Could you check a few things on this model? Use its own coordinates, in mm. A direction names the side the tool comes from. Give positions to 0.01 mm unless a question says otherwise; leave off trailing zeros. Loops run counter-clockwise (first coordinate to the right, second up) from the corner with the lowest first, then second, coordinate; pieces in that order, holes last. Notation, with made-up numbers: (21.5, 30.25) - (51.5, 30.25) arc R27 ccw to (51.5, 59.25) - close; hole circle Ø8 at (3.25, 45.25). An arc over 180 degrees is marked (long way). Write each question's results on one line, items separated by ' | '. Start each with the question number.
1) On a 3-axis mill with a long thin cutter (end or side, diameter ignored), from which of +Z, -Z, +X, -X, +Y, -Y can I reach the whole of each face in a straight line? I mean faces 1 (the face through (-1.349, 4.696, -39.603)), 2 (the face through (-46.157, 4.696, -10.863)), 3 (the face through (-50.61, 3.13, 23.15)). Say none if no direction works.
2) I want a section at B-B, the plane x = -14. Write out the boundary of the cut face in (y, z) (3 decimals).
3) If we mould it in two halves opening along Z, with no side actions, what happens to faces 4 (the face through (4.415, 3.637, 35.794)), 5 (the face through (0.1, 1.59, 34.34)), 6 (the face through (34.804, 4.696, -34.533))? For each: +Z half, -Z half, draft (parallel to the pull), parting line (faces both ways), or undercut.
4) I'm going to push flat-ended pins straight in: pin 1 (2 mm diameter, centred on y = 6, z = -20, fed in from +X); pin 2 (2 mm diameter, centred on x = -50.07, z = 16.76, fed in from +Y); pin 3 (4 mm diameter, centred on y = 4.5, z = -10, fed in from -X); pin 4 (3.5 mm diameter, centred on y = 7, z = 34.5, fed in from -X). Where does each tip first touch, or does it pass through?
5) I want a section at C-C, the plane y = 4.5. Count the separate pieces of the cut face and the enclosed holes in it, and give its area (3 significant figures).
6) I want a section at A-A, the plane z = -37. Write out the boundary of the cut face in (x, y) (3 decimals), and give its area (3 significant figures).
7) If I drill on probe 1 along Z at (x, y) = (-3.5, 2.5); probe 2 along X at (y, z) = (2.5, -1.5); probe 3 along Z at (x, y) = (-18, 2.5), over which ranges is the centre line in solid material (lowest first)? Write a range as [from, to].
from build123d import *

# Parameters (mm, degrees)
BOSS_EXTRUDE1_DEPTH = 9.525
SKETCH3_R           = 1.778
BOSS_EXTRUDE2_DEPTH = 6.35
CUT_EXTRUDE1_DEPTH  = 62.992


with BuildPart() as part:
    # Sketch2 → Boss-Extrude1 (new body)
    with BuildSketch(Plane(origin=(0, 0, 0), x_dir=(1, 0, 0), z_dir=(0, 1, 0))):
        with BuildLine():
            ThreePointArc((-27.371275132, 38.745818095), (-40.973617499, 30.433742494), (-46.191603644, 15.370975839))
            ThreePointArc((-46.191603644, 15.370975839), (-46.156170212, 10.799100226), (-46.01239655, 6.229348451))
            ThreePointArc((-46.01239655, 6.229348451), (-45.554867394, -4.424369785), (-44.211253726, -15.00292108))
            ThreePointArc((-44.211253726, -15.00292108), (-36.72609395, -29.152486681), (-21.949825784, -35.308761743))
            ThreePointArc((-21.949825784, -35.308761743), (4.789142288, -35.769006094), (31.212812312, -31.649066671))
            ThreePointArc((31.212812312, -31.649066671), (41.496738573, -25.613366213), (46.788564963, -14.927609673))
            ThreePointArc((46.788564963, -14.927609673), (47.409631974, -10.227797309), (47.362149343, -5.487364219))
            ThreePointArc((47.362149343, -5.487364219), (47.025821725, 6.063769752), (45.378811544, 17.501827706))
            ThreePointArc((45.378811544, 17.501827706), (44.784036993, 21.245111147), (43.826445822, 24.912391724))
            ThreePointArc((43.826445822, 24.912391724), (36.726457071, 37.077263766), (23.883695238, 42.861502743))
            ThreePointArc((23.883695238, 42.861502743), (-1.899636761, 42.744509754), (-27.371275132, 38.745818095))
        make_face()
        with BuildLine():
            ThreePointArc((-26.686729853, 35.645166459), (-38.494719431, 28.449859817), (-43.016527849, 15.382560778))
            ThreePointArc((-43.016527849, 15.382560778), (-42.981363707, 10.840148441), (-42.837461763, 6.299879882))
            ThreePointArc((-42.837461763, 6.299879882), (-42.392238342, -4.14410464), (-41.073809227, -14.514098915))
            ThreePointArc((-41.073809227, -14.514098915), (-34.571127727, -26.820697593), (-21.709378759, -32.141660966))
            ThreePointArc((-21.709378759, -32.141660966), (4.527721192, -32.604481914), (30.456209617, -28.565533412))
            ThreePointArc((30.456209617, -28.565533412), (39.190718322, -23.430787451), (43.667641206, -14.341539963))
            ThreePointArc((43.667641206, -14.341539963), (44.243978017, -9.976676032), (44.183339256, -5.574344354))
            ThreePointArc((44.183339256, -5.574344354), (43.863792824, 5.776703787), (42.237767725, 17.015228877))
            ThreePointArc((42.237767725, 17.015228877), (41.676987361, 20.591755151), (40.755667539, 24.092781371))
            ThreePointArc((40.755667539, 24.092781371), (34.67633853, 34.650507535), (23.588863748, 39.699440682))
            ThreePointArc((23.588863748, 39.699440682), (-1.702378082, 39.575120085), (-26.686729853, 35.645166459))
        make_face(mode=Mode.SUBTRACT)
    extrude(amount=BOSS_EXTRUDE1_DEPTH)

    # Sketch3 → Boss-Extrude2 (add)
    # profile 1 of 2: a face of its own
    with BuildSketch(Plane(origin=(0, 0, 0), x_dir=(1, 0, 0), z_dir=(0, 1, 0))):
        with BuildLine():
            ThreePointArc((43.667641206, -14.341539963), (43.210882804, -16.338608318), (42.526004307, -18.269372853))
            Line((42.526004307, -18.269372853), (61.233464192, -17.288956425))
            Line((61.233464192, -17.288956425), (60.568797548, -4.606361333))
            Line((60.568797548, -4.606361333), (44.173733451, -5.465590234))
            ThreePointArc((44.173733451, -5.465590234), (44.247134499, -9.922178586), (43.667641206, -14.341539963))
        make_face()
        with Locations(Location((51.389184551, -11.446158862, 0), (0, 0, 270))):
            Circle(SKETCH3_R, mode=Mode.SUBTRACT)
    # profile 2 of 2: a face of its own
    with BuildSketch(Plane(origin=(0, 0, 0), x_dir=(1, 0, 0), z_dir=(0, 1, 0))):
        with BuildLine():
            Line((-59.91585582, -10.920694454), (-59.251189176, -23.603289546))
            Line((-59.251189176, -23.603289546), (-38.172742485, -22.498614964))
            ThreePointArc((-38.172742485, -22.498614964), (-40.010730071, -18.741588452), (-41.048292167, -14.689809648))
            ThreePointArc((-41.048292167, -14.689809648), (-41.491708705, -12.342684149), (-41.760500894, -9.96921262))
            Line((-41.760500894, -9.96921262), (-59.91585582, -10.920694454))
        make_face()
        with Locations(Location((-50.07157618, -16.763492017, 0), (0, 0, 270))):
            Circle(SKETCH3_R, mode=Mode.SUBTRACT)
    extrude(amount=BOSS_EXTRUDE2_DEPTH)

    # Sketch4 → Cut-Extrude1 (cut)
    with BuildSketch(Plane.XY):
        with BuildLine():
            Line((-4.7625, 9.525), (4.7625, 9.525))
            Line((4.7625, 9.525), (4.7625, 6.35))
            ThreePointArc((4.7625, 6.35), (0, 1.5875), (-4.7625, 6.35))
            Line((-4.7625, 6.35), (-4.7625, 9.525))
        make_face()
    extrude(amount=CUT_EXTRUDE1_DEPTH, mode=Mode.SUBTRACT)


solid = part.part
Answers:
1) face 1: +Y, -Y | face 2: -X, +Y, -Y | face 3: +Z, +Y, -Y
2) outline: (0, -41.337) - (9.525, -41.337) - (9.525, -38.124) - (0, -38.124) - close; (0, 32.747) - (9.525, 32.747) - (9.525, 35.927) - (0, 35.927) - close
3) face 4: +Z half | face 5: draft | face 6: undercut
4) pin 1: stops at x = 45.19 | pin 2: passes through | pin 3: stops at x = -46.18 | pin 4: stops at x = -31.53
5) separate pieces: 1 | enclosed holes: 2 | area: 1,230 mm2
6) outline: (-32.614, 0) - (-20.404, 0) - (-20.404, 9.525) - (-32.614, 9.525) - close; (31.513, 0) - (36.812, 0) - (36.812, 9.525) - (31.513, 9.525) - close | area: 167 mm2
7) probe 1: z = [-42.61, -39.42], [32.94, 36.12] | probe 2: x = [-45.92, -42.74], [44.14, 47.32] | probe 3: z = [-40.68, -37.45], [32.48, 35.67]
